Autodesk Inventor part; units mm, degrees
ref_plane "YZ Plane" through (0, 0, 0) normal (1, 0, 0) x (0, 1, 0)
ref_plane "XZ Plane" through (0, 0, 0) normal (0, 1, 0) x (-1, 0, 0)
ref_plane "XY Plane" through (0, 0, 0) normal (0, 0, 1) x (1, 0, 0)
sketch "Sketch1" plane through (0, 0, 0) normal (0, 0, 1) x (1, 0, 0)
  line L0 (56.3662, 12.7852) -> (56.3662, 35.7852)
  line L1 (56.3662, 35.7852) -> (15.3628, 35.7852)
  line L2 (15.3628, 35.7852) -> (15.3662, 38.7852)
  line L3 (15.3662, 38.7852) -> (59.3662, 38.7852)
  line L4 (59.3662, 38.7852) -> (59.3662, 12.7852)
  line L5 (56.3662, 12.7852) -> (59.3662, 12.7852)
  point P0 (0, 0)
  dimension "d0" = 3
  dimension "d1" = 3
  dimension "d2" = 26
  dimension "d3" = 44
extrude "Extrusion1" add sketch "Sketch1" along normal blind 5.6
sketch "Sketch2" plane through (56.3662, 12.7852, 0) normal (-1, 0, 0) x (0, 0, 1)
  circle A0 centre (2.8, 19.3) radius 1.35
  circle A1 centre (2.8, 2.3) radius 1.35
  circle A2 centre (2.8, 19.3) radius 1.35
  circle A3 centre (2.8, 2.3) radius 1.35
  point P0 (0, -12.7852)
  dimension "d6" = 2.7
  dimension "d7" = 2.7
extrude "Extrusion2" cut sketch "Sketch2" against normal through all
sketch "Sketch3" plane through (15.3628, 35.7852, 0) normal (0, -1, 0) x (1, 0, 0)
  circle A0 centre (3.9023, 2.8) radius 1.35
  circle A1 centre (20.9023, 2.8) radius 1.35
  circle A2 centre (3.9023, 2.8) radius 1.35
  circle A3 centre (20.9023, 2.8) radius 1.35
  point P0 (-15.3628, 0)
  dimension "d10" = 2.7
  dimension "d11" = 2.7
extrude "Extrusion3" cut sketch "Sketch3" against normal through all
properties part number "Pelvis" material "Aluminum-6061"
Work out the finished part from the listing and answer in its coordinate system (mm). A direction names the side the tool comes from. Round coordinates to 2 decimals unless told otherwise and drop trailing zeros. Loops run counter-clockwise (first coordinate to the right, second up) from the corner with the lowest first, then second, coordinate; pieces in that order, holes last. Notation, with made-up numbers: M -23,2 L 18,2 A21 ccw 18,26 Z; hole C 16.25,22 d8. An arc over 180 degrees is marked long. One line per question, with ' | ' between items.
Q1. Consider line 1 along Y through (x, z) = (58.85, 2.8); line 2 along X through (y, z) = (36.75, 2.9); line 3 along Y through (x, z) = (47.5, 2.8). Determine where each line is inside the solid, lowest interval first. Write a range as from..to.
Conclusion:
line 1: y = 12.79..13.74, 16.44..30.74, 33.44..38.79 | line 2: x = 15.36..17.92, 20.61..34.92, 37.61..59.37 | line 3: y = 35.79..38.79
Q2. Find section D-D, the plane x = 46.5. Give the vertices of the cut face in (y, z), then the cut area to 3 significant figures.
Conclusion:
outline: M 35.79,0 L 38.79,0 L 38.79,5.6 L 35.79,5.6 Z | area: 16.8 mm2
Q3. Each of these flat-tipped pins is pushed along its axis until it touches: pin 1 Ø2 at (x, y) = (54, 23) entering from -Z; pin 2 Ø1.7 at (y, z) = (21.5, 3) entering from -X; pin 3 Ø1.7 at (x, z) = (42, 3) entering from -Y. Where does it stop, or does it pass through?
Conclusion:
pin 1: passes through | pin 2: stops at x = 56.37 | pin 3: stops at y = 35.79
Q4. Find section A-A, the plane z = 2.8. Give the vertices of the cut face in (x, y), then the cut area to 3 significant figures.
Conclusion:
outline: M 15.36,35.79 L 17.92,35.79 L 17.92,38.79 L 15.37,38.79 Z; M 20.62,35.79 L 34.92,35.79 L 34.92,38.79 L 20.62,38.79 Z; M 37.62,35.79 L 56.37,35.79 L 56.37,33.44 L 59.37,33.44 L 59.37,38.79 L 37.62,38.79 Z; M 56.37,12.79 L 59.37,12.79 L 59.37,13.74 L 56.37,13.74 Z; M 56.37,16.44 L 59.37,16.44 L 59.37,30.74 L 56.37,30.74 Z | area: 169 mm2
Q5. Find section B-B, the plane y = 31.25. Give the vertices of the cut face in (x, z), then the cut area to 3 significant figures.
Conclusion:
outline: M 56.37,0 L 59.37,0 L 59.37,1.74 L 56.37,1.74 Z; M 56.37,3.86 L 59.37,3.86 L 59.37,5.6 L 56.37,5.6 Z | area: 10.4 mm2
Q6. A tool of negligible diameter and unlimited length cuts with its end or side. For faces 4 (the flat face through (56.366, 24, 3)), 5 (the cylindrical face through (17.916, 37.264, 2.859)), from which of +Z, -Z, +X, -X, +Y, -Y can it reach the whole face along a straight path? Write none if from no direction.
Conclusion:
face 4: +Z, -Z, -X, -Y | face 5: +Y, -Y
Q7. The mould has two halves that part along X. Classify faces 1 (the cylindrical face through (37.55, 37.26, 3.21)), 2 (the flat face through (36, 35.785, 5)), 3 (the flat face through (59.366, 26, 3)): +X half, -X half, draft (parallel to the pull), parting line (faces both ways), or undercut.
Conclusion:
face 1: undercut | face 2: draft | face 3: +X half
Q8. Find section C-C, the plane y = 23.5. Give the vertices of the cut face in (x, z).
Conclusion:
outline: M 56.37,0 L 59.37,0 L 59.37,5.6 L 56.37,5.6 Z
